from build123d import *

# Parameters (mm, degrees)
F0_W     = 500
F0_H     = 80
F1_DEPTH = 18
F2_R     = 17.99999


# Not quite as in the source:
# - a fillet or chamfer is up to 0.001 mm smaller than in the source, because OpenCascade refuses the exact size


with BuildPart() as f1:
    # F0 (on Front) → F1 (new body)
    with BuildSketch(Plane.XZ):
        with Locations((48.9213317633, -38.1839564443)):
            Rectangle(F0_W, F0_H)
    extrude(amount=F1_DEPTH)

    # F2 (radius 18 in the source; OpenCascade refuses exactly that, so slightly less here)
    f2_edges = [f1.edges().sort_by_distance(p)[0] for p in [
        (48.921332, 0, -78.183956),
        (48.921332, 0, 1.816044),
    ]]
    fillet(f2_edges, radius=F2_R)


solid = f1.part
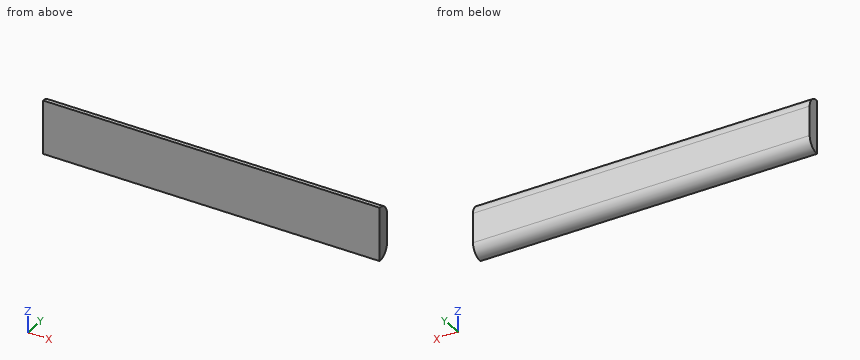
Design review of the part built by this model. Coordinates are the model's own, in mm. Round coordinates to 2 decimals unless told otherwise and drop trailing zeros. Order: outer loops, then holes, each group sorted by start corner. A loop starts at its lowest first (then second) coordinate and runs counter-clockwise, first axis right, second up.
1) Clearance check with flat-ended pins moving along their axes: pin 1 Ø1 at (x, z) = (-53.5, -64.5) entering from +Y; pin 2 Ø1.5 at (x, y) = (88, -6) entering from -Z; pin 3 Ø2 at (x, z) = (-17.5, -66) entering from +Y. State where each tip first meets the part, or that it passes through.
The answers:
pin 1: stops at y = -0.41
pin 2: stops at z = -74.24
pin 3: stops at y = -0.66
2) For L1, parallel to Y at x = 161, z = -62; L2, parallel to Z at x = 245.5, y = -17; L3, parallel to Z at x = 52, y = -15.5, list the stretches that pass through material, from the lowest coordinate up.
The answers:
L1: y = -18 to -0.09
L2: z = -78.16 to 1.79
L3: z = -78.01 to 1.64
3) Consider section B-B (y = -5). State the section outline as (x, z) points.
The answers:
outline: (-201.08, -72.63) - (298.92, -72.63) - (298.92, -3.73) - (-201.08, -3.73) - close
4) Consider section C-C (z = -3). State the section outline as (x, y) points.
The answers:
outline: (-201.08, -18) - (298.92, -18) - (298.92, -5.75) - (-201.08, -5.75) - close
